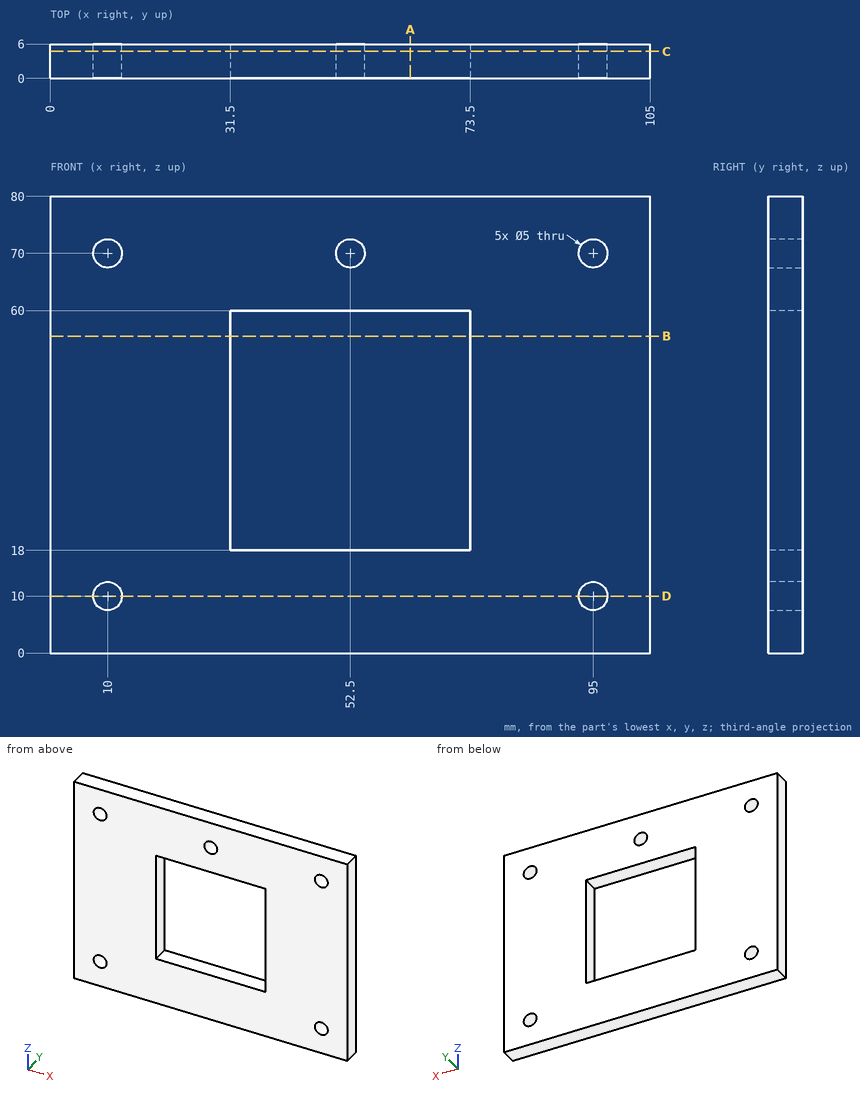
Job drawing, mm, ordinate dimensions from the low corner. One solid piece. Coordinates: 2 decimals unless noted, no trailing zeros. Write each loop counter-clockwise with the first axis right and the second up, starting at its lowest first coordinate (ties: lowest second). Pieces come first, ordered by that corner, then holes.
Item 1: Slice it at A-A (x = 63). Write the cut outline in (y, z), and give its area (3 significant figures).
Item 2: Slice it at B-B (z = 55.5). Write the cut outline in (x, y), and give its area (3 significant figures).
Item 3: Slice it at D-D (z = 10). Write the cut outline in (x, y).
Item 4: Probe line 1 (X direction, y = 4.6, z = 70); line 2 (Z direction, x = 95, y = 1.4); line 3 (X direction, y = 2.6, z = 40). List the from-to ranges inside material, lowest first.
Item 5: Slice it at C-C (y = 4.7). Write the cut outline in (x, z).
Item 6: Pin check, flat tips, straight feed: pin 1 (2 mm diameter, centred on y = 3.5, z = 35, fed in from -X); pin 2 (4 mm diameter, centred on x = 10, z = 70, fed in from -Y). Stop position of each tip, or through.
Results found:
1. outline: (0, 0) - (6, 0) - (6, 18) - (0, 18) - close; (0, 60) - (6, 60) - (6, 80) - (0, 80) - close
1. area: 228 mm2
2. outline: (0, 0) - (31.5, 0) - (31.5, 6) - (0, 6) - close; (73.5, 0) - (105, 0) - (105, 6) - (73.5, 6) - close
2. area: 378 mm2
3. outline: (0, 0) - (7.5, 0) - (7.5, 6) - (0, 6) - close; (12.5, 0) - (92.5, 0) - (92.5, 6) - (12.5, 6) - close; (97.5, 0) - (105, 0) - (105, 6) - (97.5, 6) - close
4. line 1: x = 0 to 7.5, 12.5 to 50, 55 to 92.5, 97.5 to 105
4. line 2: z = 0 to 7.5, 12.5 to 67.5, 72.5 to 80
4. line 3: x = 0 to 31.5, 73.5 to 105
5. outline: (0, 0) - (105, 0) - (105, 80) - (0, 80) - close; hole circle Ø5 at (10, 10); hole circle Ø5 at (10, 70); hole (31.5, 18) - (73.5, 18) - (73.5, 60) - (31.5, 60) - close; hole circle Ø5 at (52.5, 70); hole circle Ø5 at (95, 10); hole circle Ø5 at (95, 70)
6. pin 1: stops at x = 0
6. pin 2: passes through
